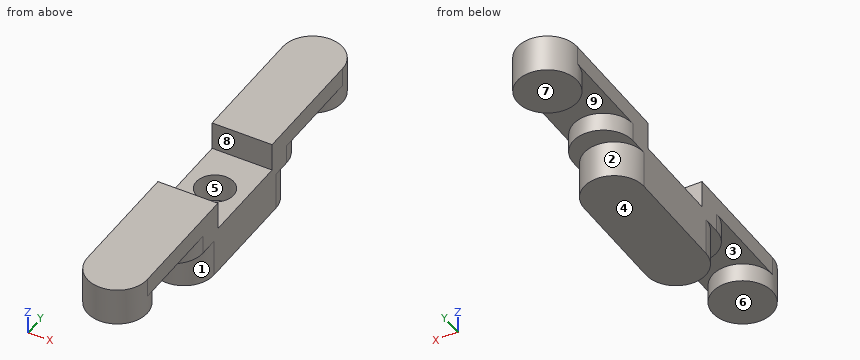
Autodesk Inventor part; units mm, degrees
ref_plane "YZ Plane" through (0, 0, 0) normal (1, 0, 0) x (0, 1, 0)
ref_plane "XZ Plane" through (0, 0, 0) normal (0, 1, 0) x (-1, 0, 0)
ref_plane "XY Plane" through (0, 0, 0) normal (0, 0, 1) x (1, 0, 0)
sketch "Sketch1" plane through (0, 0, 0) normal (0, 0, 1) x (1, 0, 0)
  line L0 (-2.31, 0) -> (2.31, 0) construction
  line L1 (0, 14.84) -> (0, -14.84) construction
  line L2 (0, 2.85) -> (0, -2.85) construction
  line L3 (-1.6, 2.85) -> (-1.6, -2.85)
  line L4 (1.6, -2.85) -> (1.6, 2.85)
  arc A0 (1.6, 2.85) -> (-1.6, 2.85) centre (0, 2.85) ccw
  arc A1 (-1.6, -2.85) -> (1.6, -2.85) centre (0, -2.85) ccw
  circle A2 centre (0, 0) radius 1
  line L5 (-1.6, 2.85) -> (-1.6, 9)
  arc A3 (1.6, 9) -> (-1.6, 9) centre (0, 9) ccw
  line L6 (1.6, 9) -> (1.6, 2.85)
  line L7 (-1.6, 2.85) -> (-1.6, 3.5)
  line L8 (1.6, 2.85) -> (1.6, 3.5)
  arc A4 (-1.6, 9) -> (1.6, 9) centre (0, 9) ccw
  line L9 (-1.6, -2.85) -> (-1.6, -9)
  arc A5 (-1.6, -9) -> (1.6, -9) centre (0, -9) ccw
  line L10 (1.6, -9) -> (1.6, -2.85)
  line L11 (-1.6, -2.85) -> (-1.6, -3.5)
  line L12 (1.6, -2.85) -> (1.6, -3.5)
  arc A6 (1.6, -9) -> (-1.6, -9) centre (0, -9) ccw
  line L13 (-1.6, 2.5) -> (1.6, 2.5)
  line L14 (-1.6, -2.5) -> (1.6, -2.5)
  arc A7 (-1.6, -3.85) -> (1.6, -3.85) centre (0, -3.85) ccw
  arc A8 (1.6, 3.85) -> (-1.6, 3.85) centre (0, 3.85) ccw
  point P0 (0, 4.45)
  point P1 (0, -4.45)
  point P2 (1.65, -3)
  point P3 (1.6008, -3)
  point P4 (-1.6008, -3)
  point P5 (-1.65, -3)
  point P6 (1.6, -2.85)
  point P7 (-1.6, -2.85)
  point P8 (-1.65, 3)
  point P9 (-1.6008, 3)
  point P10 (1.6008, 3)
  point P11 (1.65, 3)
  dimension "d2" = 2
  dimension "d16" = 2.5
  dimension "d17" = 8.9
  dimension "d18" = 3.2
  dimension "d22" = 1
extrude "Extrusion1" add sketch "Sketch1" along normal blind 1 contours A0 L4 L13 L3 | L13 L4 L14 L3 | L14 L4 A1 L3 | A2
extrude "Extrusion2" add sketch "Sketch1" along normal blind 1.5 from surface at 1 contours A0 L4 L13 L3 | L13 L4 L14 L3 | L14 L4 A1 L3
extrude "Extrusion3" add sketch "Sketch1" along normal blind 0.5 from surface at 2.5 contours A0 L4 L13 L3 | L14 L4 A1 L3
extrude "Extrusion4" add sketch "Sketch1" along normal blind 1 from surface at 3 contours A0 L4 L13 L3 | L5 A8 L6 A0 | L14 L4 A1 L3 | L5 A4 L6 A8 | A1 L10 A7 L9 | A3 A4 | A7 L10 A6 L9 | A6 A5
extrude "Extrusion5" add sketch "Sketch1" against normal blind 1 from surface at 3 contours A3 A4 | A6 A5
extrude "Extrusion6" add sketch "Sketch1" against normal blind 1 from surface at 3 contours L5 A8 L6 A0 | A1 L10 A7 L9
properties part number "Button Cap"
Verification items for the finished model (mm, model axes). Face numbers are marked on the shaded views. A direction names the side the tool comes from. Coordinates: 2 decimals unless noted, no trailing zeros. Order: outer loops, then holes, each group sorted by start corner. A loop starts at its lowest first (then second) coordinate and runs counter-clockwise, first axis right, second up. Notation, with made-up numbers: (13.5, 2) -> (35.5, 2) arc R37 ccw to (35.5, 41) -> close; hole circle Ø3 at (-29, 78.25). An arc over 180 degrees is marked (long way). Put each result on its own line as item: value. Start each with the question number.
1. Material ranges on L1, parallel to Y at x = 0, z = 1.55; L2, parallel to Y at x = -0.75, z = 2.35; L3, parallel to Z at x = 0.5, y = -1.25, recorded low to high. Write a range as [from, to].
2. Access from +Z, -Z, +X, -X, +Y, -Y to the whole of each face (thin tool, end or side, straight path). Record for the marked faces 5, 6, 7, 8 and 9.
3. Cross-section at A-A, the plane z = 3.2. Record the boundary of the cut face in (x, y), then the cut area to 3 significant figures.
4. Cross-section at D-D, the plane y = 5.25. Record the boundary of the cut face in (x, z).
5. Mould release check, pull along Y, two halves, no side actions. Record for the marked faces 1, 2, 3 and 4: released by +Y, released by -Y, zero draft, split by the parting line, or undercut.
6. Cross-section at C-C, the plane x = -0.3. Record the boundary of the cut face in (y, z).
7. Cross-section at B-B, the plane y = 8. Record the boundary of the cut face in (x, z).
8. Go/stop test with flat-tipped pins: pin 1 Ø1.6 at (x, y) = (-0.5, 9.5) entering from -Z; pin 2 Ø1.6 at (x, y) = (0, 0) entering from +Z. Record where each tip stops, or that it passes through.
Computed:
1. L1: [-4.45, -1], [1, 4.45]
1. L2: [-10.41, -7.59], [-5.26, -0.66], [0.66, 5.26], [7.59, 10.41]
1. L3: [0, 2.5]
2. face 5: +Z
2. face 6: -Z, +X, -X, -Y
2. face 7: -Z, +X, -X, +Y
2. face 8: +Z, +X, -X
2. face 9: -Z
3. outline: (-1.6, -9) arc R1.6 ccw to (1.6, -9) -> (1.6, -2.5) -> (-1.6, -2.5) -> close; (-1.6, 2.5) -> (1.6, 2.5) -> (1.6, 9) arc R1.6 ccw to (-1.6, 9) -> close
3. area: 49.6 mm2
4. outline: (-1.6, 3) -> (-0.77, 3) -> (-0.77, 2) -> (0.77, 2) -> (0.77, 3) -> (1.6, 3) -> (1.6, 4) -> (-1.6, 4) -> close
5. face 1: released by -Y
5. face 2: released by +Y
5. face 3: undercut
5. face 4: zero draft
6. outline: (-10.57, 2) -> (-7.43, 2) -> (-7.43, 3) -> (-5.42, 3) -> (-5.42, 2) -> (-4.42, 2) -> (-4.42, 0) -> (4.42, 0) -> (4.42, 2) -> (5.42, 2) -> (5.42, 3) -> (7.43, 3) -> (7.43, 2) -> (10.57, 2) -> (10.57, 4) -> (2.5, 4) -> (2.5, 2.5) -> (0.95, 2.5) -> (0.95, 1) -> (-0.95, 1) -> (-0.95, 2.5) -> (-2.5, 2.5) -> (-2.5, 4) -> (-10.57, 4) -> close
7. outline: (-1.6, 3) -> (-1.25, 3) -> (-1.25, 2) -> (1.25, 2) -> (1.25, 3) -> (1.6, 3) -> (1.6, 4) -> (-1.6, 4) -> close
8. pin 1: z = 2
8. pin 2: z = 1
